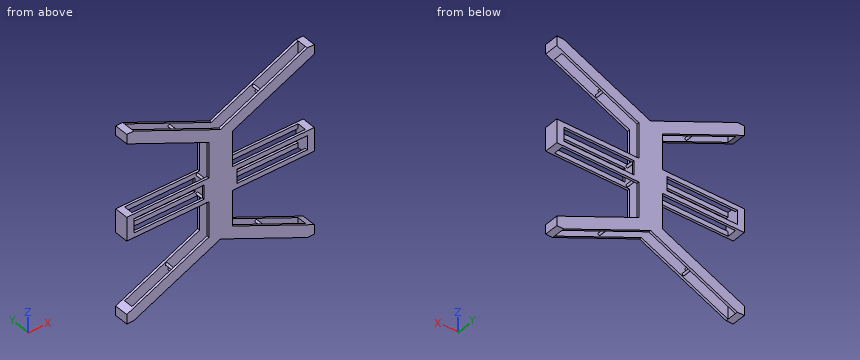
from build123d import *

# Parameters (mm, degrees)
BOSS_EXTRUDE1_DEPTH      = 6
BOSS_EXTRUDE1_DEPTH_BACK = 6
SKETCH2_W                = 148
SKETCH2_H                = 8
CUT_EXTRUDE1_DEPTH       = 160
SKETCH4_W                = 60
SKETCH4_H                = 12
CUT_EXTRUDE2_DEPTH       = 12
SKETCH5_R                = 1
BOSS_EXTRUDE2_DEPTH      = 8


with BuildPart() as part:
    # Sketch1 → Boss-Extrude1 (new, two sides: drawn at the far end of the back side and taken through both)
    with BuildSketch(Plane(origin=(0, 0, 0), x_dir=(1, 0, 0), z_dir=(0, 1, 0)).offset(-BOSS_EXTRUDE1_DEPTH_BACK)):
        Polygon((80, 10), (80, -10), (10, -10), (10, -40), (80, -72), (80, -80), (74, -80), (0, -46.171428571), (-74, -80), (-80, -80), (-80, -72), (-10, -40), (-10, -10), (-80, -10), (-80, 10), (-10, 10), (-10, 40), (-80, 72), (-80, 80), (-74, 80), (0, 46.171428571), (74, 80), (80, 80), (80, 72), (10, 40), (10, 10), align=None)
    extrude(amount=BOSS_EXTRUDE1_DEPTH + BOSS_EXTRUDE1_DEPTH_BACK)

    # Sketch2 → Cut-Extrude1 (cut)
    with BuildSketch(Plane.XY.offset(80)):
        Rectangle(SKETCH2_W, SKETCH2_H)
    extrude(amount=-CUT_EXTRUDE1_DEPTH, mode=Mode.SUBTRACT)

    # Sketch4 → Cut-Extrude2 (cut)
    with BuildSketch(Plane(origin=(0, 6, 0), x_dir=(1, 0, 0), z_dir=(0, 1, 0))):
        with Locations((-44, 0)):
            Rectangle(SKETCH4_W, SKETCH4_H)
        with Locations((44, 0)):
            Rectangle(SKETCH4_W, SKETCH4_H)
    extrude(amount=-CUT_EXTRUDE2_DEPTH, mode=Mode.SUBTRACT)

    # Sketch5 → Boss-Extrude2 (add)
    with BuildSketch(Plane(origin=(0, -4, 0), x_dir=(1, 0, 0), z_dir=(0, 1, 0))):
        with Locations(Location((-35.87258255, -60.371251291, 0), (0, 0, 90))):
            Circle(SKETCH5_R)
        with Locations(Location((-38.271663698, -55.12326128, 0), (0, 0, 90))):
            Circle(SKETCH5_R)
        with Locations(Location((-12, -8, 0), (0, 0, 90))):
            Circle(SKETCH5_R)
        with Locations(Location((0, -40.171428571, 0), (0, 0, 90))):
            Circle(SKETCH5_R)
        with Locations(Location((12, -8, 0), (0, 0, 90))):
            Circle(SKETCH5_R)
        with Locations(Location((35.87258255, -60.371251291, 0), (0, 0, 90))):
            Circle(SKETCH5_R)
        with Locations(Location((38.271663698, -55.12326128, 0), (0, 0, 90))):
            Circle(SKETCH5_R)
        with Locations(Location((38.271663698, 55.12326128, 0), (0, 0, 90))):
            Circle(SKETCH5_R)
        with Locations(Location((35.87258255, 60.371251291, 0), (0, 0, 90))):
            Circle(SKETCH5_R)
        with Locations(Location((-35.87258255, 60.371251291, 0), (0, 0, 90))):
            Circle(SKETCH5_R)
        with Locations(Location((-38.271663698, 55.12326128, 0), (0, 0, 90))):
            Circle(SKETCH5_R)
        with Locations(Location((0, 40.171428571, 0), (0, 0, 90))):
            Circle(SKETCH5_R)
        with Locations(Location((12, 8, 0), (0, 0, 90))):
            Circle(SKETCH5_R)
        with Locations(Location((-12, 8, 0), (0, 0, 90))):
            Circle(SKETCH5_R)
    extrude(amount=BOSS_EXTRUDE2_DEPTH)


solid = part.part
Input: part model. Units: mm. Frame: model coordinates. Give positions to 0.01 mm unless a question says otherwise; leave off trailing zeros. Loops run counter-clockwise (first coordinate to the right, second up) from the corner with the lowest first, then second, coordinate; pieces in that order, holes last. Notation, with made-up numbers: (18, 35.5) - (47, 35.5) arc R34 ccw to (47, 69.5) - close; hole circle Ø5 at (69.5, 69.5). An arc over 180 degrees is marked (long way). Use CSV: the item, a comma, the result in double quotes. Start each with the question number.
Item 1: Contact query for flat-ended pins moving along their axis: P1, Ø2, axis at y = 4.5, z = 20, coming from the -X side; P2, Ø2, axis at x = 39, y = 5, coming from the +Z side; P3, Ø1, axis at y = 4, z = 63.5, coming from the +X side. Output: stop coordinate, or through.
Item 2: Section A-A on z = -27. Return loops of the section in (x, y), then the cut area to 3 significant figures.
Item 3: Line query: line 1 (Z direction, x = -35.5, y = -4.25); line 2 (Z direction, x = 71, y = 5.75); line 3 (Y direction, x = -2, z = 13). Output: solid intervals per line, ascending.
Item 4: Section B-B on x = -19. State how many separate pieces and enclosed holes the cut face has, then the cut area to 3 significant figures.
Ans:
1,P1,"stops at x = -10"
1,P2,"stops at z = 64.46"
1,P3,"stops at x = 62.5"
2,outline,"(-10, -6) - (10, -6) - (10, -4) - (-10, -4) - close; (-10, 4) - (10, 4) - (10, 6) - (-10, 6) - close"
2,area,"80.0 mm2"
3,line 1,"z = -62.4 to -51.66, -10 to -6, 6 to 10, 51.66 to 62.4"
3,line 2,"z = -78.63 to -67.89, -10 to -6, 6 to 10, 67.89 to 78.63"
3,line 3,"y = -6 to -4, 4 to 6"
4,separate pieces,"8"
4,enclosed holes,"0"
4,area,"118 mm2"
